from build123d import *

# Parameters (mm, degrees)
F1_DEPTH = 2.54


with BuildPart() as f1:
    # F0 (on Top) → F1 (new body)
    with BuildSketch(Plane.XY):
        with BuildLine():
            ThreePointArc((-8.43737, 5.660069), (0, 10.16), (8.43737, 5.660069))
            ThreePointArc((8.43737, 5.660069), (13.036176, 1.503456), (19.05, 0))
            Line((19.05, 0), (19.05, 2.54))
            ThreePointArc((19.05, 2.54), (14.231471, 3.744632), (10.546713, 7.075087))
            ThreePointArc((10.546713, 7.075087), (0, 12.7), (-10.546713, 7.075087))
            ThreePointArc((-10.546713, 7.075087), (-14.231471, 3.744632), (-19.05, 2.54))
            Line((-19.05, 2.54), (-19.05, 0))
            ThreePointArc((-19.05, 0), (-13.036176, 1.503456), (-8.43737, 5.660069))
        make_face()
    extrude(amount=F1_DEPTH)


solid = f1.part
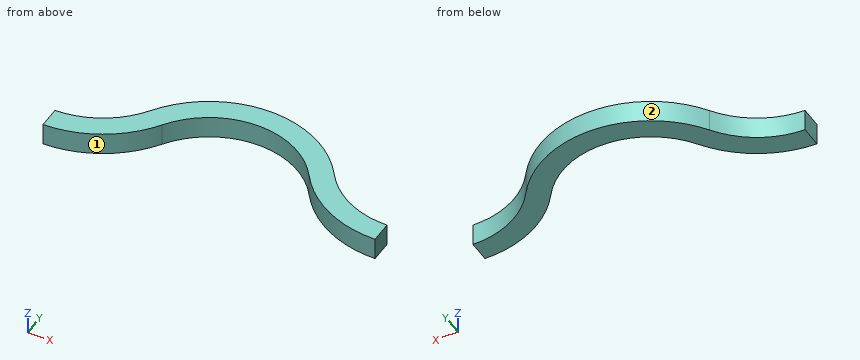
Geometry: final body of the model. Coordinates: model frame, mm. Face numbers are marked on the shaded views. A direction names the side the tool comes from. Coordinates: 2 decimals unless noted, no trailing zeros. Loops run counter-clockwise (first coordinate to the right, second up) from the corner with the lowest first, then second, coordinate; pieces in that order, holes last. Notation, with made-up numbers: (74.5, 31) - (118.5, 31) arc R21 cw to (118.5, 53) - close; hole circle Ø7 at (-8, 43.5). An arc over 180 degrees is marked (long way). One line per question, with ' | ' between items. Start each with the question number.
(1) Ray query, L1, parallel to X at y = 8.5, z = 2; L2, parallel to X at y = 6, z = 1.45; L3, parallel to Y at x = -3, z = 0.25. Return the intervals inside material, ascending. Write a range as from..to.
(2) Cut plane A-A on y = 3.5. Output: boundary loops of the cut face in (x, z), and give its area (3 significant figures).
(3) Cut plane D-D on x = 5. Output: boundary loops of the cut face in (y, z).
(4) Cut plane B-B on z = 0.9. Output: boundary loops of the cut face in (x, y), and give its area (3 significant figures).
(5) Reachability of the marked faces 1 and 2 from +Z, -Z, +X, -X, +Y, -Y: full face, straight path, thin tool, end or side. Return the list, or none.
(6) Cut plane C-C on y = 6.25. Output: boundary loops of the cut face in (x, z).
Here are the results:
1) L1: -9.44..-5.57, 5.57..9.44 | L2: -11.38..-8.2, 8.2..11.38 | L3: 9.71..12.34
2) outline: (-14.72, 0) - (-10.26, 0) - (-10.26, 2.54) - (-14.72, 2.54) - close; (10.26, 0) - (14.72, 0) - (14.72, 2.54) - (10.26, 2.54) - close | area: 22.6 mm²
3) outline: (8.84, 0) - (11.67, 0) - (11.67, 2.54) - (8.84, 2.54) - close
4) outline: (-19.05, 0) arc R12.78 ccw to (-8.44, 5.66) arc R10.16 cw to (8.44, 5.66) arc R12.78 ccw to (19.05, 0) - (19.05, 2.54) arc R10.24 cw to (10.55, 7.08) arc R12.7 ccw to (-10.55, 7.08) arc R10.24 cw to (-19.05, 2.54) - close | area: 114 mm²
5) face 1: +Z, -Z, -Y | face 2: +Z, -Z, +Y
6) outline: (-11.16, 0) - (-8.01, 0) - (-8.01, 2.54) - (-11.16, 2.54) - close; (8.01, 0) - (11.16, 0) - (11.16, 2.54) - (8.01, 2.54) - close
